from build123d import *

# Parameters (mm, degrees)
BOSS_EXTRUDE1_DEPTH = 0.2
SKETCH3_R           = 5
BOSS_EXTRUDE2_DEPTH = 0.2
SKETCH4_R           = 5
CUT_EXTRUDE1_DEPTH  = 0.05
FILLET1_R           = 0.5
FILLET2_R           = 0.2


with BuildPart() as part:
    # Sketch2 → Boss-Extrude1 (new body)
    with BuildSketch(Plane.XY):
        with BuildLine():
            Line((-5.123848106, -13.5), (5.123848106, -13.5))
            ThreePointArc((5.123848106, -13.5), (5.830954887, -13.207106781), (6.123848106, -12.5))
            Line((6.123848106, -12.5), (6.123848106, -8.39885311))
            ThreePointArc((6.123848106, -8.39885311), (6.155941006, -8.042003499), (6.251189751, -7.696606227))
            Line((6.251189751, -7.696606227), (7.872658355, -3.372689949))
            ThreePointArc((7.872658355, -3.372689949), (7.9679071, -3.027292676), (8, -2.670443065))
            Line((8, -2.670443065), (8, 12.5))
            ThreePointArc((8, 12.5), (7.707106781, 13.207106781), (7, 13.5))
            Line((7, 13.5), (-7, 13.5))
            ThreePointArc((-7, 13.5), (-7.707106781, 13.207106781), (-8, 12.5))
            Line((-8, 12.5), (-8, -2.670443065))
            ThreePointArc((-8, -2.670443065), (-7.9679071, -3.027292676), (-7.872658355, -3.372689949))
            Line((-7.872658355, -3.372689949), (-6.251189751, -7.696606227))
            ThreePointArc((-6.251189751, -7.696606227), (-6.155941006, -8.042003499), (-6.123848106, -8.39885311))
            Line((-6.123848106, -8.39885311), (-6.123848106, -12.5))
            ThreePointArc((-6.123848106, -12.5), (-5.830954887, -13.207106781), (-5.123848106, -13.5))
        make_face()
    extrude(amount=BOSS_EXTRUDE1_DEPTH)

    # Sketch3 → Boss-Extrude2 (add)
    with BuildSketch(Plane(origin=(0, 0, 0), x_dir=(-1, 0, 0), z_dir=(0, 0, -1))):
        with BuildLine():
            Line((1, 0.098294397), (1, -13.875268119))
            Line((1, -13.875268119), (1.189324579, -13.875268119))
            ThreePointArc((1.189324579, -13.875268119), (1.401456614, -13.963136085), (1.489324579, -14.175268119))
            Line((1.489324579, -14.175268119), (1.489324579, -15.850374766))
            Line((1.489324579, -15.850374766), (2.110675421, -15.850374766))
            Line((2.110675421, -15.850374766), (2.110675421, -14.175268119))
            ThreePointArc((2.110675421, -14.175268119), (2.198543386, -13.963136085), (2.410675421, -13.875268119))
            Line((2.410675421, -13.875268119), (2.6, -13.875268119))
            Line((2.6, -13.875268119), (2.6, 0.588618902))
            ThreePointArc((2.6, 0.588618902), (0, 12.417117813), (-2.6, 0.588618902))
            Line((-2.6, 0.588618902), (-2.6, -13.875268119))
            Line((-2.6, -13.875268119), (-2.410675421, -13.875268119))
            ThreePointArc((-2.410675421, -13.875268119), (-2.198543386, -13.963136085), (-2.110675421, -14.175268119))
            Line((-2.110675421, -14.175268119), (-2.110675421, -15.850374766))
            Line((-2.110675421, -15.850374766), (-1.489324579, -15.850374766))
            Line((-1.489324579, -15.850374766), (-1.489324579, -14.175268119))
            ThreePointArc((-1.489324579, -14.175268119), (-1.401456614, -13.963136085), (-1.189324579, -13.875268119))
            Line((-1.189324579, -13.875268119), (-1, -13.875268119))
            Line((-1, -13.875268119), (-1, 0.098294397))
            ThreePointArc((-1, 0.098294397), (0, 0.017117813), (1, 0.098294397))
        make_face()
        with Locations((0, 6.217117813)):
            Circle(SKETCH3_R, mode=Mode.SUBTRACT)
    extrude(amount=-BOSS_EXTRUDE2_DEPTH)

    # Sketch4 → Cut-Extrude1 (cut)
    with BuildSketch(Plane(origin=(0, 0, 0), x_dir=(-1, 0, 0), z_dir=(0, 0, -1))):
        with BuildLine():
            Line((1, -13.875268119), (1.189324579, -13.875268119))
            ThreePointArc((1.189324579, -13.875268119), (1.401456614, -13.963136085), (1.489324579, -14.175268119))
            Line((1.489324579, -14.175268119), (1.489324579, -15.850374766))
            Line((1.489324579, -15.850374766), (2.110675421, -15.850374766))
            Line((2.110675421, -15.850374766), (2.110675421, -14.175268119))
            ThreePointArc((2.110675421, -14.175268119), (2.198543386, -13.963136085), (2.410675421, -13.875268119))
            Line((2.410675421, -13.875268119), (2.6, -13.875268119))
            Line((2.6, -13.875268119), (2.6, 0.588618902))
            ThreePointArc((2.6, 0.588618902), (0, 12.417117813), (-2.6, 0.588618902))
            Line((-2.6, 0.588618902), (-2.6, -13.875268119))
            Line((-2.6, -13.875268119), (-2.410675421, -13.875268119))
            ThreePointArc((-2.410675421, -13.875268119), (-2.198543386, -13.963136085), (-2.110675421, -14.175268119))
            Line((-2.110675421, -14.175268119), (-2.110675421, -15.850374766))
            Line((-2.110675421, -15.850374766), (-1.489324579, -15.850374766))
            Line((-1.489324579, -15.850374766), (-1.489324579, -14.175268119))
            ThreePointArc((-1.489324579, -14.175268119), (-1.401456614, -13.963136085), (-1.189324579, -13.875268119))
            Line((-1.189324579, -13.875268119), (-1, -13.875268119))
            Line((-1, -13.875268119), (-1, 0.098294397))
            ThreePointArc((-1, 0.098294397), (0, 0.017117813), (1, 0.098294397))
            Line((1, 0.098294397), (1, -13.875268119))
        make_face()
        with Locations((0, 6.217117813)):
            Circle(SKETCH4_R, mode=Mode.SUBTRACT)
    extrude(amount=-CUT_EXTRUDE1_DEPTH, mode=Mode.SUBTRACT)

    # Fillet1
    # the kernel refuses this fillet: 0.5 mm, written as the material it takes off along each edge
    with BuildSketch(Plane(origin=(-2.6, -13.875268119, -0.888170298), x_dir=(0, 1, 0), z_dir=(0, 0, 1)), Plane(origin=(1, -13.875268119, -0.888170298), x_dir=(0, 1, 0), z_dir=(0, 0, 1))) as fillet1_piece_1:
        with BuildLine():
            CenterArc((0.438912275, -0.49593288), FILLET1_R, 97.312922169, 60.15129319)
            Line((-0.022907897, -0.304302692), (-0.069089914, -0.285139673))
            ThreePointArc((-0.069089914, -0.285139673), (-0.05, -0.189324579), (-0.05, 0))
            Line((-0.05, 0), (0, 0.05))
            ThreePointArc((0, 0.05), (0.18763406, 0.05), (0.368903703, 0.049593288))
            Line((0.368903703, 0.049593288), (0.375268119, 0))
        make_face()
    extrude(amount=2.026340595, mode=Mode.SUBTRACT)
    with BuildSketch(Plane(origin=(-1, -13.875268119, -0.888170298), x_dir=(-0.997178450014068, -0.07506756175300172, 0), z_dir=(0, 0, 1)), Plane(origin=(2.6, -13.875268119, -0.888170298), x_dir=(-0.997178450014068, -0.07506756175300161, 0), z_dir=(0, 0, 1))) as fillet1_piece_2:
        with BuildLine():
            CenterArc((0.461585506, -0.474902334), FILLET1_R, 108.23068039, 60.15129319)
            Line((-0.028170463, -0.374209281), (-0.07714606, -0.364139976))
            ThreePointArc((-0.07714606, -0.364139976), (-0.063944154, -0.183351263), (-0.049858923, 0.003753378))
            Line((-0.049858923, 0.003753378), (0.003753378, 0.049858923))
            ThreePointArc((0.003753378, 0.049858923), (0.192543769, 0.035646788), (0.289521549, 0.047490233))
            Line((0.289521549, 0.047490233), (0.305163727, 0))
        make_face()
    extrude(amount=2.026340595, mode=Mode.SUBTRACT)

    # Fillet2
    fillet2_edges = [part.edges().sort_by_distance(p)[0] for p in [
        (-2.110675421, -15.850374766, 0.125),
        (-1.489324579, -15.850374766, 0.125),
        (1.489324579, -15.850374766, 0.125),
        (2.110675421, -15.850374766, 0.125),
    ]]
    fillet(fillet2_edges, radius=FILLET2_R)


solid = part.part
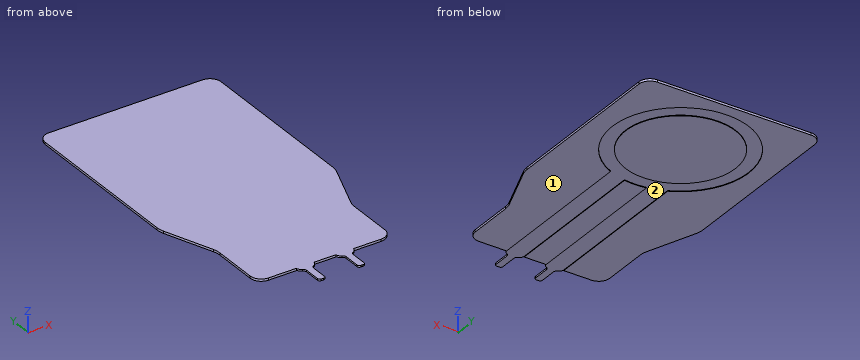
Geometry check sheet. Reference: the model listing, model coordinates, mm. Face numbers are marked on the shaded views. Round coordinates to 2 decimals unless told otherwise and drop trailing zeros. Order: outer loops, then holes, each group sorted by start corner. A loop starts at its lowest first (then second) coordinate and runs counter-clockwise, first axis right, second up. Notation, with made-up numbers: M 50.5,-9.75 L 54.5,-9.75 A23 ccw 54.5,28.25 Z; hole C 85,27.5 d4. An arc over 180 degrees is marked long. Write each question's results on one line, items separated by ' | '. Start each with the question number.
1. Material ranges on L1, parallel to Y at x = 4.25, z = 0.15; L2, parallel to Z at x = -1.75, y = -2.75; L3, parallel to X at y = -13.75, z = 0.1, recorded low to high. Write a range as from..to.
2. Cross-section at A-A on x = 0. Record the boundary of the cut face in (y, z).
3. Cross-section at B-B on y = -13. Record the boundary of the cut face in (x, z).
4. Draft check along Y on the marked faces 1 and 2. Enter one of: pulls with the +Y half, pulls with the -Y half, needs draft (parallel to the pull), parting line crosses it, or undercut.
Resolved:
1) L1: -13.5..13.5 | L2: 0.05..0.2 | L3: -2.49..-1.11, 1.11..2.49
2) outline: M -13.5,0 L 0.02,0 L 0.02,0.05 L 1.22,0.05 L 1.22,0 L 11.22,0 L 11.22,0.05 L 12.42,0.05 L 12.42,0 L 13.5,0 L 13.5,0.2 L -13.5,0.2 Z
3) outline: M -5.99,0 L -2.6,0 L -2.6,0.05 L -1,0.05 L -1,0 L 1,0 L 1,0.05 L 2.6,0.05 L 2.6,0 L 5.99,0 L 5.99,0.2 L -5.99,0.2 Z
4) face 1: needs draft | face 2: undercut
